```python
from build123d import *

# Parameters (mm, degrees)
F0_W    = 10
F0_H    = 2
F0_W_2  = 20
F0_H_2  = 8.5
F2_SIZE = 1


with BuildPart() as f1:
    # F0 (on Top) → F1 (revolve)
    with BuildSketch(Plane.XY):
        with BuildLine():
            Line((0, 2), (0, 0))
            Line((0, 0), (150, 0))
            Line((150, 0), (150, 10))
            ThreePointArc((150, 10), (147.071068, 17.071068), (140, 20))
            Line((140, 20), (10, 20))
            ThreePointArc((10, 20), (2.928932, 17.071068), (0, 10))
            Line((0, 10), (0, 2))
        make_face()
        with Locations((-5, 1)):
            Rectangle(F0_W, F0_H)
        Polygon((-60, 0), (-10, 0), (-10, 2), (-10, 10), (-60, 10), (-60, 8.5), align=None)
        with Locations((-70, 4.25)):
            Rectangle(F0_W_2, F0_H_2)
    revolve(axis=Axis((-35, 0, 0), (-1, 0, 0)))

    # F2
    f2_edges = [f1.edges().sort_by_distance(p)[0] for p in [
        (-80, -8.5, 0),
    ]]
    chamfer(f2_edges, length=F2_SIZE)


solid = f1.part
```
Input: part model. Units: mm. Frame: model coordinates. A direction names the side the tool comes from. Give positions to 0.01 mm unless a question says otherwise; leave off trailing zeros. Order: outer loops, then holes, each group sorted by start corner. A loop starts at its lowest first (then second) coordinate and runs counter-clockwise, first axis right, second up.
1. Material intervals for L1, parallel to X at y = -4, z = -8.5; L2, parallel to X at y = 3.5, z = -5.5; L3, parallel to Z at x = 133.5, y = 0.5, sorted ascending.
Derived:
L1: x = -60 to -10, 0 to 150
L2: x = -80 to -10, 0 to 150
L3: z = -19.99 to 19.99
2. Pin query (flat end, axial travel): pin 1 (3 mm diameter, centred on x = 122.5, z = 15, fed in from -Y); pin 2 (4 mm diameter, centred on y = 7.5, z = 13.5, fed in from -X); pin 3 (1.5 mm diameter, centred on x = 83, y = -14.5, fed in from +Z). Return the tip coordinate at first contact, or that it passes through.
Derived:
pin 1: stops at y = -14.76
pin 2: stops at x = 0.61
pin 3: stops at z = 14.52
3. Mould query, pull axis X, two halves, no side actions, for faces 3 (the cylindrical face through (-5, 0, 2)), 4 (the cylindrical face through (-35.35, -2.17, 9.76)), 5 (the flat face through (-10, 0.1, -2.4)), 6 (the flat face through (150, 0, 0)). Classes: released by +X, released by -X, zero draft, split by the parting line, or undercut.
Derived:
face 3: undercut
face 4: zero draft
face 5: undercut
face 6: released by +X
4. Section A-A on y = 0. Return the cut outline in (x, z).
Derived:
outline: (-80, -7.5) - (-79, -8.5) - (-60, -8.5) - (-60, -10) - (-10, -10) - (-10, -2) - (0, -2) - (0, -10) arc R10 ccw to (10, -20) - (140, -20) arc R10 ccw to (150, -10) - (150, 10) arc R10 ccw to (140, 20) - (10, 20) arc R10 ccw to (0, 10) - (0, 2) - (-10, 2) - (-10, 10) - (-60, 10) - (-60, 8.5) - (-79, 8.5) - (-80, 7.5) - close
5. Reachability of faces 1 (the cylindrical face through (-69.367, 4.57, -7.167)), 2 (the cylindrical face through (74.09, -4.336, 19.524)) from +Z, -Z, +X, -X, +Y, -Y: full face, straight path, thin tool, end or side. Return the list, or none.
Derived:
face 1: -X
face 2: +X, -X
6. Section C-C on x = 19. Return the cut outline in (y, z).
Derived:
outline: circle Ø40 at (0, 0)
